from build123d import *

# Parameters (mm, degrees)
SKETCH_1_R          = 4
EXTRUDE_1_DEPTH     = 1.25
CUT_EXTRUDE_1_DEPTH = 22
EXTRUDE_START       = -2.5
EXTRUDE_2_DEPTH     = 2.5
CUT_EXTRUDE_START   = -2.5
CUT_EXTRUDE_2_DEPTH = 2.5
CUT_EXTRUDE_4_DEPTH = 10
FILLET_1_R          = 4


with BuildPart() as part:
    # 草图1 → 凸台-拉伸1 (new, symmetric)
    with BuildSketch(Plane.XY):
        with BuildLine():
            Line((-1.233702436, 4.84540796), (14.292269552, 8.798517714))
            Line((14.292269552, 8.798517714), (27.541816671, 8.302545362))
            Line((27.541816671, 8.302545362), (50.285691672, 7.168894271))
            Line((50.285691672, 7.168894271), (48.971743891, -1.387225717))
            Line((48.971743891, -1.387225717), (38.114277377, -2.724152564))
            Line((38.114277377, -2.724152564), (18.384478153, -4.790312237))
            Line((18.384478153, -4.790312237), (3.124153733, -7.364758207))
            Line((3.124153733, -7.364758207), (-2.372822781, -4.401103504))
            ThreePointArc((-2.372822781, -4.401103504), (-4.962484216, 0.611351292), (-1.233702436, 4.84540796))
        make_face()
        Circle(SKETCH_1_R, mode=Mode.SUBTRACT)
    extrude(amount=EXTRUDE_1_DEPTH, both=True)

    # 草图2 → 切除-拉伸1 (cut)
    with BuildSketch(Plane.XY.offset(1.25)):
        with BuildLine():
            ThreePointArc((6, -2.05), (26.381158068, -1.352479883), (46.666940766, 0.736816365))
            ThreePointArc((46.666940766, 0.736816365), (47.563889378, 1.920236488), (46.380469254, 2.8171851))
            ThreePointArc((46.380469254, 2.8171851), (26.237586384, 0.742606553), (6, 0.05))
            ThreePointArc((6, 0.05), (4.95, -1), (6, -2.05))
        make_face()
    extrude(amount=-CUT_EXTRUDE_1_DEPTH, mode=Mode.SUBTRACT)

    # 草图3 → 凸台-拉伸2 (add)
    with BuildSketch(Plane(origin=(0, 0, -1.25), x_dir=(-1, 0, 0), z_dir=(0, 0, -1)).offset(EXTRUDE_START)):
        with BuildLine():
            Line((3.830222216, -3.213938048), (-2.597653881, -10.87438248))
            ThreePointArc((-2.597653881, -10.87438248), (-25.103045153, -6.203517484), (-48.061011216, -7.317703438))
            Line((-48.061011216, -7.317703438), (-48.971743891, -1.387225717))
            Line((-48.971743891, -1.387225717), (-38.114277377, -2.724152564))
            Line((-38.114277377, -2.724152564), (-18.384478153, -4.790312237))
            Line((-18.384478153, -4.790312237), (-3.124153733, -7.364758207))
            Line((-3.124153733, -7.364758207), (2.372822781, -4.401103504))
            ThreePointArc((2.372822781, -4.401103504), (3.157812892, -3.876624529), (3.830222216, -3.213938048))
        make_face()
    extrude(amount=EXTRUDE_2_DEPTH)

    # 草图4 → 切除-拉伸2 (cut)
    with BuildSketch(Plane(origin=(0, 0, -1.25), x_dir=(-1, 0, 0), z_dir=(0, 0, -1)).offset(CUT_EXTRUDE_START)):
        with BuildLine():
            Line((-48.675283939, -3.317703438), (-38.061011216, -6.114773366))
            ThreePointArc((-38.061011216, -6.114773366), (-43.07765861, -6.577848026), (-48.061011216, -7.317703438))
            Line((-48.061011216, -7.317703438), (-48.675283939, -3.317703438))
        make_face()
    extrude(amount=CUT_EXTRUDE_2_DEPTH, mode=Mode.SUBTRACT)

    # 草图6 → 切除-拉伸4 (cut)
    with BuildSketch(Plane(origin=(0, 0, -1.25), x_dir=(-1, 0, 0), z_dir=(0, 0, -1))):
        with BuildLine():
            ThreePointArc((-21.916565225, -6.331777176), (-20.02762746, -6.571548728), (-18.144467787, -6.853126294))
            ThreePointArc((-18.144467787, -6.853126294), (-10.276894061, -8.499690713), (-2.597653881, -10.87438248))
            Line((-2.597653881, -10.87438248), (-0.832664521, -8.770950068))
            Line((-0.832664521, -8.770950068), (-21.916565225, -6.331777176))
        make_face()
    extrude(amount=-CUT_EXTRUDE_4_DEPTH, mode=Mode.SUBTRACT)

    # 圆角1
    fillet_1_edges = [part.edges().sort_by_distance(p)[0] for p in [
        (14.292269552, 8.798517714, 0),
        (27.541816671, 8.302545362, 0),
        (50.285691672, 7.168894271, 0),
        (48.675283939, -3.317703438, 0),
        (38.061011216, -6.114773366, 0),
        (0.832664521, -8.770950068, 0),
    ]]
    fillet(fillet_1_edges, radius=FILLET_1_R)


solid = part.part
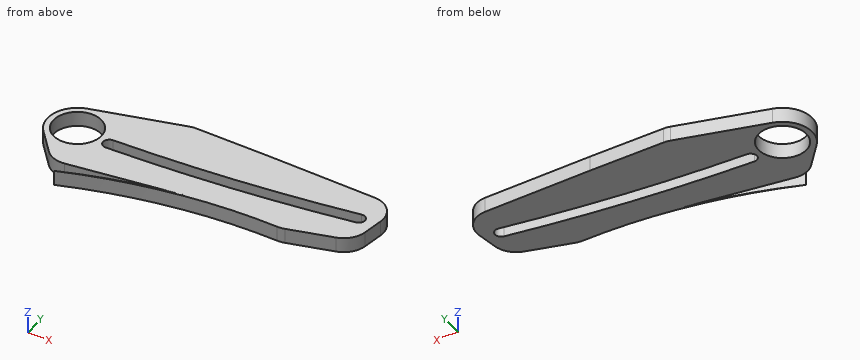
Check sheet for the modelled part. Datum: model origin and axes. Units: mm. Round coordinates to 2 decimals unless told otherwise and drop trailing zeros. Order: outer loops, then holes, each group sorted by start corner. A loop starts at its lowest first (then second) coordinate and runs counter-clockwise, first axis right, second up.
Q1. Cross-section at C-C, the plane x = 16.5. Enter the section's corners in (y, z).
Filled sheet:
outline: (-7.29, -1.25) - (-7.13, -1.25) - (-7.13, 1.25) - (-7.29, 1.25) - close; (-6.96, -1.25) - (-1.87, -1.25) - (-1.87, 1.25) - (-6.96, 1.25) - close; (0.24, -1.25) - (8.72, -1.25) - (8.72, 1.25) - (0.24, 1.25) - close
Q2. Cross-section at B-B, the plane x = 43. Enter the section's corners in (y, z), plus the area to 3 significant figures.
Filled sheet:
outline: (-4.81, -1.25) - (0.26, -1.25) - (0.26, 1.25) - (-4.81, 1.25) - close; (2.37, -1.25) - (7.53, -1.25) - (7.53, 1.25) - (2.37, 1.25) - close
area: 25.6 mm2
Q3. Cross-section at D-D, the plane z = 0.3. Give the number of separate pieces and of enclosed holes in the cut face, plus the area to 3 significant figures.
Filled sheet:
separate pieces: 1
enclosed holes: 2
area: 600 mm2
Q4. Cross-section at A-A, the plane y = 1.75. Enter the section's corners in (x, z), plus the area to 3 significant figures.
Filled sheet:
outline: (-4.68, -1.25) - (-3.6, -1.25) - (-3.6, 1.25) - (-4.68, 1.25) - close; (3.6, -1.25) - (37.68, -1.25) - (37.68, 1.25) - (3.6, 1.25) - close; (47.57, -1.25) - (49.45, -1.25) - (49.45, 1.25) - (47.57, 1.25) - close
area: 92.6 mm2
Q5. Scan lines: L1, parallel to Y at x = 24, z = 0.5; L2, parallel to Y at x = 45, z = -0.8; L3, parallel to X at y = -3.25, z = 1.15. Record each from-to range of solid material in increasing order.
Filled sheet:
L1: y = -6.3 to -1.51, 0.6 to 8.44
L2: y = -4.29 to 0.51, 2.63 to 7.43
L3: x = -3.8 to -2.33, 2.33 to 47.61
Q6. Depth check by flat-ended pin: P1, Ø1, axis at x = 12.5, z = 1, coming from the +Y side. Enter the tip coordinate at first touch or a pass-through.
Filled sheet:
P1: stops at y = 8.47
